from build123d import *

# Parameters (mm, degrees)
F1_DEPTH = 2.5
F2_DEPTH = 123.5
F3_W     = 6
F3_H     = 19
F4_DEPTH = 8
F6_D     = 3
F6_DEPTH = 5
F6_TIP   = 0.9012909285
F5_W     = 5
F5_H     = 12
F7_DEPTH = 25.5
F8_START = 20
F5_W_2   = 20
F8_DEPTH = 5.5
F9_R     = 1


with BuildPart() as f1:
    # F0 (on Top) → F1 (new body)
    with BuildSketch(Plane.XY):
        Polygon((10, 31), (1, 40), (-1, 40), (-10, 31), (-10, -31), (-1, -40), (1, -40), (10, -31), align=None)
    extrude(amount=F1_DEPTH)

    # F0 (on Top) → F2 (join)
    with BuildSketch(Plane.XY):
        Polygon((12.500000447, -32.0355340911), (12.500000447, 32.0355340911), (2.0355340911, 42.500000447), (-2.0355340911, 42.500000447), (-12.500000447, 32.0355340911), (-12.500000447, -32.0355340911), (-2.0355340911, -42.500000447), (2.0355340911, -42.500000447), align=None)
        Polygon((-1, 40), (1, 40), (10, 31), (10, -31), (1, -40), (-1, -40), (-10, -31), (-10, 31), align=None, mode=Mode.SUBTRACT)
    extrude(amount=F2_DEPTH)

    # F3 (on face) → F4 (cut)
    with BuildSketch(Plane(origin=(0, 0, 0), x_dir=(1, 0, 0), z_dir=(0, 0, -1))):
        with Locations((9.500000447, 15.5355340911)):
            Rectangle(F3_W, F3_H)
    extrude(amount=-F4_DEPTH, mode=Mode.SUBTRACT)

    # F6
    with Locations(Plane.YZ.offset(12.500000447)):
        with Locations((13.5, 18.25)):
            Hole(F6_D / 2, depth=F6_DEPTH)
            with Locations((0, 0, -(F6_DEPTH + F6_TIP / 2))):  # 118° drill point
                Cone(0, F6_D / 2, F6_TIP, mode=Mode.SUBTRACT)

    # F5 (on face) → F7 (join)
    with BuildSketch(Plane.YZ.offset(12.500000447)):
        with Locations((2.5, 90.5)):
            Rectangle(F5_W, F5_H)
    extrude(amount=F7_DEPTH)

    # F5 (on face) → F8 (join)
    with BuildSketch(Plane.YZ.offset(12.500000447).offset(F8_START)):
        with Locations((15, 90.5)):
            Rectangle(F5_W_2, F5_H)
    extrude(amount=F8_DEPTH)

    # F9
    f9_edges = [f1.edges().sort_by_distance(p)[0] for p in [
        (12.5, 0, 123.5),
        (7.267767, 37.267767, 123.5),
        (0, 42.5, 123.5),
        (-7.267767, 37.267767, 123.5),
        (-12.5, 0, 123.5),
        (-7.267767, -37.267767, 123.5),
        (0, -42.5, 123.5),
        (7.267767, -37.267767, 123.5),
        (0, 40, 123.5),
        (5.5, 35.5, 123.5),
        (10, 0, 123.5),
        (5.5, -35.5, 123.5),
        (0, -40, 123.5),
        (-5.5, -35.5, 123.5),
        (-10, 0, 123.5),
        (-5.5, 35.5, 123.5),
        (22.5, 5, 96.5),
        (32.5, 15, 96.5),
        (35.25, 25, 96.5),
        (38, 12.5, 96.5),
        (25.25, 0, 96.5),
        (12.5, 2.5, 96.5),
        (25.25, 0, 84.5),
        (38, 12.5, 84.5),
        (35.25, 25, 84.5),
        (32.5, 15, 84.5),
        (22.5, 5, 84.5),
        (12.5, 2.5, 84.5),
        (7.267767, -37.267767, 0),
        (0, -42.5, 0),
        (-7.267767, -37.267767, 0),
        (-12.5, 0, 0),
        (-7.267767, 37.267767, 0),
        (0, 42.5, 0),
        (7.267767, 37.267767, 0),
        (12.5, 13, 0),
        (9.5, -6.035534, 0),
        (6.5, -15.535534, 0),
        (9.5, -25.035534, 0),
        (12.5, -28.535534, 0),
        (-2.035534, 42.5, 61.75),
        (-12.5, 32.035534, 61.75),
        (-12.5, -32.035534, 61.75),
        (-2.035534, -42.5, 61.75),
        (2.035534, 42.5, 61.75),
        (12.5, 32.035534, 61.75),
        (12.5, -32.035534, 61.75),
        (2.035534, -42.5, 61.75),
        (11.25, -6.035534, 8),
        (10, -15.535534, 8),
        (11.25, -25.035534, 8),
        (12.5, -15.535534, 8),
        (6.5, -15.535534, 2.5),
        (32.5, 25, 90.5),
        (38, 25, 90.5),
        (38, 0, 90.5),
        (10, -25.035534, 5.25),
        (12.5, -25.035534, 4),
        (10, -6.035534, 5.25),
        (12.5, -6.035534, 4),
        (12.5, 5, 90.5),
        (12.5, 0, 90.5),
    ]]
    fillet(f9_edges, radius=F9_R)


solid = f1.part
The listing builds one solid part. Answer for the finished solid, in the listing's coordinates (mm). A direction names the side the tool comes from. Give positions to 0.01 mm unless a question says otherwise; leave off trailing zeros. Loops run counter-clockwise (first coordinate to the right, second up) from the corner with the lowest first, then second, coordinate; pieces in that order, holes last. Notation, with made-up numbers: (77, 1) - (132, 1) arc R21 ccw to (132, 7) - close; hole circle Ø7 at (73, -18). An arc over 180 degrees is marked (long way). Answer as a JSON object with one key per item and string values.
1. Flat-ended cylindrical pins translate along their axes: pin 1 Ø5 at (x, z) = (7, 49) entering from -Y; pin 2 Ø1 at (x, z) = (35, 91.5) entering from +Y; pin 3 Ø7 at (x, y) = (25, 7) entering from +Z. Find the tip coordinate at first contact, or state that the pin passes through.
Determined:
{"pin 1": "y = -40.04", "pin 2": "y = 25", "pin 3": "z = 96.5"}
2. Find the intervals of material crossed by L1, parallel to X at y = 8, z = 93; L2, parallel to X at y = 21, z = 64.5; L3, parallel to X at y = -35.5, z = 98, in increasing order. Write a range as [from, to].
Determined:
{"L1": "[-12.5, -10], [10, 12.5], [32.5, 38]", "L2": "[-12.5, -10], [10, 12.5]", "L3": "[-9.04, -5.5], [5.5, 9.04]"}
3. For faces 4 (the flat face through (-7.199, 37.337, 60.899)), 5 (the flat face through (23, 5, 90)), 6 (the flat face through (5, 36, 62)), determine the directions among +Z, -Z, +X, -X, +Y, -Y from which every point of the face is accessible in a straight line to the end or side of a thin tool.
Determined:
{"face 4": "+Z, -Z, -X, +Y", "face 5": "+Z, -Z, +Y", "face 6": "+Z"}
4. A cutting plane is placed at C-C (z = 31). Write down the section's boundary in (x, y).
Determined:
{"outline": "(-12.5, -31.62) arc R1 ccw to (-12.21, -32.33) - (-2.33, -42.21) arc R1 ccw to (-1.62, -42.5) - (1.62, -42.5) arc R1 ccw to (2.33, -42.21) - (12.21, -32.33) arc R1 ccw to (12.5, -31.62) - (12.5, 31.62) arc R1 ccw to (12.21, 32.33) - (2.33, 42.21) arc R1 ccw to (1.62, 42.5) - (-1.62, 42.5) arc R1 ccw to (-2.33, 42.21) - (-12.21, 32.33) arc R1 ccw to (-12.5, 31.62) - close; hole (-10, -31) - (-1, -40) - (1, -40) - (10, -31) - (10, 31) - (1, 40) - (-1, 40) - (-10, 31) - close"}
5. A cutting plane is placed at A-A (y = 8.5). Write down the section's boundary in (x, z), then the cut area to 3 significant figures.
Determined:
{"outline": "(-12.5, 1) arc R1 ccw to (-11.5, 0) - (11.5, 0) arc R1 ccw to (12.5, 1) - (12.5, 122.5) arc R1 ccw to (11.5, 123.5) - (11, 123.5) arc R1 ccw to (10, 122.5) - (10, 2.5) - (-10, 2.5) - (-10, 122.5) arc R1 ccw to (-11, 123.5) - (-11.5, 123.5) arc R1 ccw to (-12.5, 122.5) - close; (32.5, 85.5) arc R1 ccw to (33.5, 84.5) - (37, 84.5) arc R1 ccw to (38, 85.5) - (38, 95.5) arc R1 ccw to (37, 96.5) - (33.5, 96.5) arc R1 ccw to (32.5, 95.5) - close", "area": "731 mm²"}
6. A cutting plane is placed at D-D (x = 16.5). Write down the section's boundary in (y, z).
Determined:
{"outline": "(0, 85.5) arc R1 ccw to (1, 84.5) - (4, 84.5) arc R1 ccw to (5, 85.5) - (5, 95.5) arc R1 ccw to (4, 96.5) - (1, 96.5) arc R1 ccw to (0, 95.5) - close"}
7. For a pull along Y with two mould halves and no side action, classify faces 1 (the flat face through (34, 8, 84.5)), 2 (the flat face through (-6, 35, 62)), 3 (the flat face through (-7.337, -37.199, 60.899)) as pulls with the +Y half, pulls with the -Y half, needs draft (parallel to the pull), parting line crosses it, or undercut.
Determined:
{"face 1": "needs draft", "face 2": "undercut", "face 3": "pulls with the -Y half"}
8. A cutting plane is placed at B-B (z = 18.25). Write down the section's boundary in (x, y).
Determined:
{"outline": "(-12.5, -31.62) arc R1 ccw to (-12.21, -32.33) - (-2.33, -42.21) arc R1 ccw to (-1.62, -42.5) - (1.62, -42.5) arc R1 ccw to (2.33, -42.21) - (12.21, -32.33) arc R1 ccw to (12.5, -31.62) - (12.5, 12) - (10, 12) - (10, -31) - (1, -40) - (-1, -40) - (-10, -31) - (-10, 31) - (-1, 40) - (1, 40) - (10, 31) - (10, 15) - (12.5, 15) - (12.5, 31.62) arc R1 ccw to (12.21, 32.33) - (2.33, 42.21) arc R1 ccw to (1.62, 42.5) - (-1.62, 42.5) arc R1 ccw to (-2.33, 42.21) - (-12.21, 32.33) arc R1 ccw to (-12.5, 31.62) - close"}
